from build123d import *


with BuildPart() as part:
    # Sketch1 → Revolve1 (revolve)
    with BuildSketch(Plane.XY, mode=Mode.PRIVATE) as revolve1_sk:
        with BuildLine():
            Line((0, 0), (31.75, 0))
            Line((31.75, 0), (31.75, 3.175))
            Line((31.75, 3.175), (25.4, 3.175))
            Line((25.4, 3.175), (25.4, 6.35))
            Line((25.4, 6.35), (21.95, 6.35))
            ThreePointArc((21.95, 6.35), (8.479615818, 11.929615818), (2.9, 25.4))
            Line((2.9, 25.4), (2.9, 57.15))
            Line((2.9, 57.15), (0, 57.15))
            Line((0, 57.15), (0, 0))
        make_face()
    revolve(revolve1_sk.sketch.rotate(Axis((0, 0, 0), (0, -1, 0)), 90), axis=Axis((0, 0, 0), (0, -1, 0)))


solid = part.part
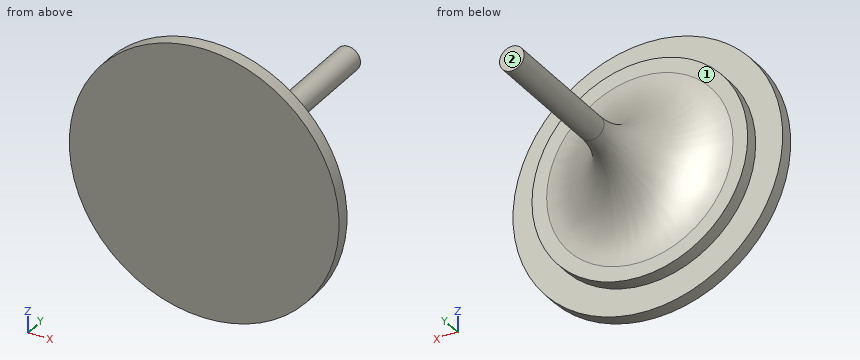
Source: CAD feature listing. Evaluate the final solid. Frame: model axes, mm. Face numbers are marked on the shaded views. A direction names the side the tool comes from. Give positions to 0.01 mm unless a question says otherwise; leave off trailing zeros. Order: outer loops, then holes, each group sorted by start corner. A loop starts at its lowest first (then second) coordinate and runs counter-clockwise, first axis right, second up. Notation, with made-up numbers: (8.5, 79.5) -> (31.5, 79.5) arc R27 cw to (31.5, 96.5) -> close; hole circle Ø5 at (28.5, 71.5). An arc over 180 degrees is marked (long way). Write item = value, one per line.
Q1. Cut plane A-A, the plane x = 0. Output: boundary loops of the cut face in (y, z) (3 decimals), and give its area (3 significant figures).
Data:
outline = (0, -31.75) -> (3.175, -31.75) -> (3.175, -25.4) -> (6.35, -25.4) -> (6.35, -21.95) arc R19.05 cw to (25.4, -2.9) -> (57.15, -2.9) -> (57.15, 2.9) -> (25.4, 2.9) arc R19.05 cw to (6.35, 21.95) -> (6.35, 25.4) -> (3.175, 25.4) -> (3.175, 31.75) -> (0, 31.75) -> close
area = 813 mm^2
Q2. Cut plane B-B, the plane z = 0. Output: boundary loops of the cut face in (x, y) (3 decimals).
Data:
outline = (-31.75, 0) -> (31.75, 0) -> (31.75, 3.175) -> (25.4, 3.175) -> (25.4, 6.35) -> (21.95, 6.35) arc R19.05 cw to (2.9, 25.4) -> (2.9, 57.15) -> (-2.9, 57.15) -> (-2.9, 25.4) arc R19.05 cw to (-21.95, 6.35) -> (-25.4, 6.35) -> (-25.4, 3.175) -> (-31.75, 3.175) -> close
Q3. Cut plane C-C, the plane y = 50. Output: boundary loops of the cut face in (x, z).
Data:
outline = circle Ø5.8 at (0, 0)
Q4. Cut plane D-D, the plane y = 11. Output: boundary loops of the cut face in (x, z).
Data:
outline = circle Ø18.96 at (0, 0)
Q5. Material intervals for line 1 (Y direction, x = 8.5, z = -26) (3 decimals); line 2 (Y direction, x = 1, z = 22.5); line 3 (X direction, y = 41, z = -0.5), sorted ascending. Write a range as from..to.
Data:
line_1 = 0..3.175
line_2 = 0..6.35
line_3 = -2.86..2.86
Q6. Set-up query: the marked faces 1 and 2. Return all of +Z, -Z, +X, -X, +Y, -Y with unobstructed straight access to the full face (end or side cutting, diameter ignored); none if empty.
Data:
face_1 = +Y
face_2 = +Z, -Z, +X, -X, +Y
Q7. Pin query (flat end, axial travel): pin 1 (6 mm diameter, centred on y = 28, z = -6.5, fed in from +X); pin 2 (8 mm diameter, centred on x = -3, y = 16, fed in from -Z); pin 3 (3 mm diameter, centred on x = 4, y = 18.5, fed in from -Z); pin 4 (12 mm diameter, centred on x = -1, y = 26, fed in from +Z). Return the tip coordinate at first contact, or that it passes through.
Data:
pin_1 = through
pin_2 = -8.04
pin_3 = -3.61
pin_4 = 3.66
